Read the model definition and answer for the solid it produces. Units are mm, in the model's axes. Face numbers are marked on the shaded views. Round coordinates to 2 decimals unless told otherwise and drop trailing zeros. Order: outer loops, then holes, each group sorted by start corner. A loop starts at its lowest first (then second) coordinate and runs counter-clockwise, first axis right, second up.
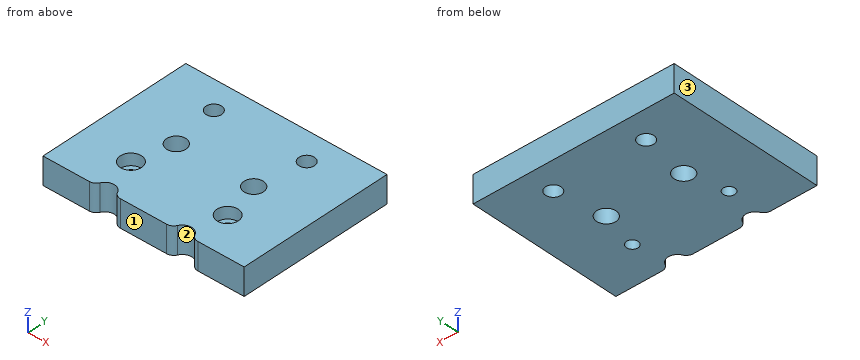
Autodesk Inventor part; units mm, degrees
ref_plane "YZ Plane" through (0, 0, 0) normal (1, 0, 0) x (0, 1, 0)
ref_plane "XZ Plane" through (0, 0, 0) normal (0, 1, 0) x (-1, 0, 0)
ref_plane "XY Plane" through (0, 0, 0) normal (0, 0, 1) x (1, 0, 0)
sketch "Boceto21" plane through (0, 0, 0) normal (0, 0, 1) x (1, 0, 0)
  line L0 (-26, 15) -> (26, 15)
  line L1 (26, 15) -> (26, -15)
  line L2 (26, -15) -> (-26, -15)
  line L3 (-26, -15) -> (-26, 15)
  line L4 (1.8793, 0) -> (0, 0)
  line L5 (0, 0) -> (0, 2.1218)
  dimension "d96" = 52
  dimension "d97" = 30
extrude "Extrusión17" add sketch "Boceto21" along normal blind 7
sketch "Boceto22" plane through (0, 0, 7) normal (0, 0, 1) x (1, 0, 0)
  circle A0 centre (-12.5, -5) radius 1.5
  circle A1 centre (12.5, -5) radius 1.5
  line L0 (-26, -15) -> (26, -15)
  point P0 (0, 0)
  dimension "d100" = 3
  dimension "d101" = 3
  dimension "d104" = 10
  dimension "d105" = 10
  dimension "d106" = 25
  dimension "d107" = 12.5
extrude "Extrusión18" cut sketch "Boceto22" against normal through all
sketch "Boceto23" plane through (0, 0, 7) normal (0, 0, 1) x (1, 0, 0)
  circle A0 centre (10, 5) radius 2.5
  circle A1 centre (10, -15) radius 2.5
  circle A2 centre (12.5, -5) radius 1.5
  point P0 (0, 0)
  dimension "d110" = 5
  dimension "d111" = 5
  dimension "d112" = 10
  dimension "d113" = 10
  dimension "d114" = 20
  dimension "d115" = 10
extrude "Extrusión19" cut sketch "Boceto23" against normal through all contours A0 | A1
mirror "Simetría1" about plane through (0, 0, 0) normal (1, 0, 0) of "Extrusión19"
fillet "Empalme5" radius 2 4 edges at (-12.5, -15, 3.5) (-7.5, -15, 3.5) (12.5, -15, 3.5) (7.5, -15, 3.5)
sketch "Boceto24" plane through (0, 0, 7) normal (0, 0, 1) x (1, 0, 0)
  circle A0 centre (12.5, -5) radius 1.5
  circle A1 centre (12.5, -5) radius 2.75
  circle A2 centre (-12.5, -5) radius 1.5
  circle A3 centre (-12.5, -5) radius 2.75
  point P0 (0, 0)
  dimension "d119" = 5.5
  dimension "d120" = 5.5
extrude "Extrusión20" cut sketch "Boceto24" against normal blind 3
sketch "Boceto25" plane through (0, 0, 7) normal (0, 0, 1) x (1, 0, 0)
  line L0 (26, 15) -> (-26, 15)
  line L1 (-26, 15) -> (-26, 25)
  line L2 (-26, 25) -> (26, 25)
  line L3 (26, 25) -> (26, 15)
  point P0 (0, 0)
  dimension "d123" = 10
extrude "Extrusión21" add sketch "Boceto25" against normal up to surface (7 mm away)
sketch "Boceto26" plane through (0, 0, 7) normal (0, 0, 1) x (1, 0, 0)
  circle A0 centre (12, 17.682) radius 2
  circle A1 centre (12.5, -5) radius 2.75
  circle A2 centre (-12, 17.682) radius 2
  circle A3 centre (-12.5, -5) radius 2.75
  circle A4 centre (10, 5) radius 2.5
  circle A5 centre (-10, 5) radius 2.5
  point P0 (0, 0)
  dimension "d127" = 12
  dimension "d128" = 4
  dimension "d129" = 4
  dimension "d132" = 12
  dimension "d135" = 12.682
  dimension "d136" = 12.682
extrude "Extrusión22" cut sketch "Boceto26" against normal through all contours A0 | A2
equation "\"d101\" = d100"
equation "\"d105\" = d104"
equation "\"d111\" = d110"
equation "\"d120\" = d119"
equation "\"d128\" = d129"
equation "\"d136\" = d135"
properties part number "Soporte Extruder Izq" material "Polipropileno"
Q1. Straight lines are drawn through the part: probe 1 along Y at (x, z) = (12, 5.25); probe 2 along X at (y, z) = (3, 4.25); probe 3 along X at (y, z) = (-5.5, 4.25). For each, find the intervals that lie inside material, in ascending order.
Outcome:
probe 1: y = -13.5 to -7.7, -2.3 to 3.5, 6.5 to 15.68, 19.68 to 25
probe 2: x = -26 to -11.5, -8.5 to 8.5, 11.5 to 26
probe 3: x = -26 to -15.2, -9.8 to 9.8, 15.2 to 26
Q2. A cutting plane is placed at B-B, the plane z = 2.75. Give the vertices of the cut face in (x, y), plus the area to 3 significant figures.
Outcome:
outline: (-26, -15) - (-14.03, -15) arc R2 ccw to (-12.24, -13.89) arc R2.5 cw to (-7.76, -13.89) arc R2 ccw to (-5.97, -15) - (5.97, -15) arc R2 ccw to (7.76, -13.89) arc R2.5 cw to (12.24, -13.89) arc R2 ccw to (14.03, -15) - (26, -15) - (26, 25) - (-26, 25) - close; hole circle Ø3 at (-12.5, -5); hole circle Ø4 at (-12, 17.68); hole circle Ø5 at (-10, 5); hole circle Ø5 at (10, 5); hole circle Ø4 at (12, 17.68); hole circle Ø3 at (12.5, -5)
area: 1,980 mm2
Q3. A cutting plane is placed at A-A, the plane y = 5. Give the vertices of the cut face in (x, z).
Outcome:
outline: (-26, 0) - (-12.5, 0) - (-12.5, 7) - (-26, 7) - close; (-7.5, 0) - (7.5, 0) - (7.5, 7) - (-7.5, 7) - close; (12.5, 0) - (26, 0) - (26, 7) - (12.5, 7) - close
Q4. For a pull along X with two mould halves and no side action, classify the marked faces 1, 2 and 3 as released by +X, released by -X, zero draft, split by the parting line, or undercut.
Outcome:
face 1: zero draft
face 2: undercut
face 3: released by -X
Q5. A cutting plane is placed at C-C, the plane z = 5.75. Give the vertices of the cut face in (x, y).
Outcome:
outline: (-26, -15) - (-14.03, -15) arc R2 ccw to (-12.24, -13.89) arc R2.5 cw to (-7.76, -13.89) arc R2 ccw to (-5.97, -15) - (5.97, -15) arc R2 ccw to (7.76, -13.89) arc R2.5 cw to (12.24, -13.89) arc R2 ccw to (14.03, -15) - (26, -15) - (26, 25) - (-26, 25) - close; hole circle Ø5.5 at (-12.5, -5); hole circle Ø4 at (-12, 17.68); hole circle Ø5 at (-10, 5); hole circle Ø5 at (10, 5); hole circle Ø5.5 at (12.5, -5); hole circle Ø4 at (12, 17.68)
Q6. A flat-ended cylindrical pin translates along its axis: pin 1 (5 mm diameter, centred on x = 12.5, y = -5, fed in from +Z). Find the tip coordinate at first contact, or state that the pin passes through.
Outcome:
pin 1: stops at z = 4
